from build123d import *

# Parameters (mm, degrees)
EXTRUDE_1_DEPTH           = 6
HOLE_WIZARD_1_D           = 3
HOLE_WIZARD_1_DEPTH       = 6
HOLE_WIZARD_1_CBORE_D     = 5
HOLE_WIZARD_1_CBORE_DEPTH = 3


with BuildPart() as part:
    # 草图1 → 凸台-拉伸1 (new body)
    with BuildSketch(Plane.XY):
        Polygon((0, 5.5), (-9.526279442, 0), (0, -5.5), (9.526279442, 0), align=None)
    extrude(amount=EXTRUDE_1_DEPTH)

    # 孔1
    with Locations(Plane(origin=(0.973720558, 0, 6), x_dir=(1, 0, 0), z_dir=(0, 0, 1))):
        with Locations((0, 0)):
            CounterBoreHole(HOLE_WIZARD_1_D / 2, HOLE_WIZARD_1_CBORE_D / 2, HOLE_WIZARD_1_CBORE_DEPTH, depth=HOLE_WIZARD_1_DEPTH)


solid = part.part
Check sheet for the modelled part. Datum: model origin and axes. Units: mm. A direction names the side the tool comes from. Round coordinates to 2 decimals unless told otherwise and drop trailing zeros. Loops run counter-clockwise (first coordinate to the right, second up) from the corner with the lowest first, then second, coordinate; pieces in that order, holes last. Notation, with made-up numbers: (10.25, 89.25) - (38.25, 89.25) arc R12 ccw to (38.25, 109.25) - close; hole circle Ø4 at (59, 6.25). An arc over 180 degrees is marked (long way). Answer as CSV lines item,"result". Start each with the question number.
Item 1: Set-up check for faces 1 (the flat face through (-2, 0, 6)), 2 (the flat face through (1, -2, 3)): record each of +Z, -Z, +X, -X, +Y, -Y from which the full face is reachable in a straight line by a thin tool's end or side.
Item 2: Section check C-C (x = 2.25). Record the boundary of the cut face in (y, z).
Item 3: Scan lines: line 1 (Y direction, x = -0.25, z = 0.8); line 2 (X direction, y = -1, z = 3.65) (3 decimals); line 3 (Y direction, x = 4, z = 4.7). Record each from-to range of solid material in increasing order. Write a range as [from, to].
Item 4: Section check D-D (y = 4). Record the boundary of the cut face in (x, z).
Item 5: Depth check by flat-ended pin: P1, Ø1.5, axis at y = 4, z = 5, coming from the +X side; P2, Ø1.5, axis at x = 2, z = 1.5, coming from the -Y side; P3, Ø5, axis at x = 6.5, y = 1.5, coming from the -Z side; P4, Ø4, axis at x = 0.97, y = 0, coming from the +Z side. Enter the tip coordinate at first touch or a pass-through.
Item 6: Section check B-B (y = 0.5). Record the boundary of the cut face in (x, z).
Item 7: Release check for a two-part mould opening along X. For faces 3 (the cylindrical face through (-0.457, 0.451, 1.479)), 4 (the flat face through (4.696, -2.788, 2.958)), 5 (the flat face through (-0.1, 1.3, 0)), 6 (the flat face through (-4.83, -2.71, 2.96)) record: +X half, -X half, draft (parallel to the pull), parting line (faces both ways), or undercut.
Item 8: Section check A-A (z = 2.2). Record the boundary of the cut face in (x, y).
Report:
1,face 1,"+Z, +X, -X, +Y, -Y"
1,face 2,"+Z"
2,outline,"(-4.2, 0) - (-0.79, 0) - (-0.79, 3) - (-2.15, 3) - (-2.15, 6) - (-4.2, 6) - close; (0.79, 0) - (4.2, 0) - (4.2, 6) - (2.15, 6) - (2.15, 3) - (0.79, 3) - close"
3,line 1,"y = [-5.36, -0.87], [0.87, 5.36]"
3,line 2,"x = [-7.794, -1.318], [3.265, 7.794]"
3,line 3,"y = [-3.19, 3.19]"
4,outline,"(-2.6, 0) - (2.6, 0) - (2.6, 6) - (-2.6, 6) - close"
5,P1,"stops at x = 3.9"
5,P2,"stops at y = -4.78"
5,P3,"stops at z = 0"
5,P4,"stops at z = 3"
6,outline,"(-8.66, 0) - (-0.44, 0) - (-0.44, 3) - (-1.48, 3) - (-1.48, 6) - (-8.66, 6) - close; (2.39, 0) - (8.66, 0) - (8.66, 6) - (3.42, 6) - (3.42, 3) - (2.39, 3) - close"
7,face 3,"undercut"
7,face 4,"+X half"
7,face 5,"draft"
7,face 6,"-X half"
8,outline,"(-9.53, 0) - (0, -5.5) - (9.53, 0) - (0, 5.5) - close; hole circle Ø3 at (0.97, 0)"
